The drawing under review shows one solid part. Ordinate dimensions are in mm from its lowest x, y, z. A direction names the side the tool comes from. Give positions to 0.01 mm unless a question says otherwise; leave off trailing zeros. Order: outer loops, then holes, each group sorted by start corner. A loop starts at its lowest first (then second) coordinate and runs counter-clockwise, first axis right, second up. Notation, with made-up numbers: (48.25, 39.25) - (62.25, 39.25) arc R22 cw to (62.25, 74.25) - close; hole circle Ø10 at (68.25, 12.25). An arc over 180 degrees is marked (long way). Answer as a JSON object with one key per item and string values. Group by question number.
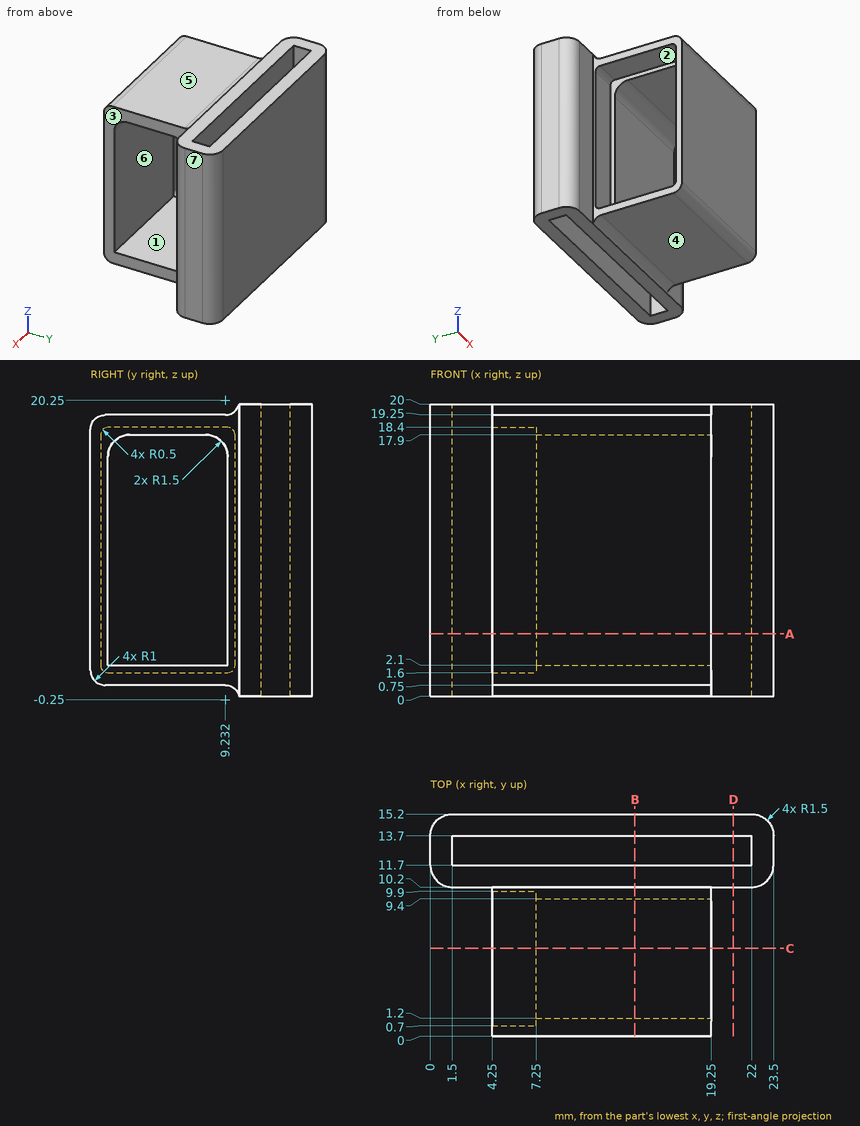
1) Consider section D-D (x = 20.75). Give the boundary of the cut face in (y, z), plus the area to 3 significant figures.
2) For line 1 (Y direction, x = 11, z = 5); line 2 (Z direction, x = 12.5, y = 3); line 3 (Y direction, x = 3, z = 16), list the stretches that pass through material, from the lowest coordinate up.
3) Consider section C-C (y = 6). Give the boundary of the cut face in (x, z), plus the area to 3 significant figures.
4) Consider section A-A (z = 4.25). Give the boundary of the cut face in (x, y), plus the area to 3 significant figures.
5) For pin 1 (8 mm diameter, centred on x = 4, y = 2, fed in from +Z); pin 2 (6 mm diameter, centred on y = 5, z = 17, fed in from -X); pin 3 (3 mm diameter, centred on x = 2.5, z = 14.5, fed in from -Y), all flat-tipped, find the tip position at first contact; note any pin that passes through.
6) Mouldability with a two-part tool opening along Z and no side actions: class the marked faces 4, 5, 6 and 7 as released by +Z, released by -Z, zero draft, split by the parting line, or undercut.
7) For the marked faces 1, 2 and 3, list the 3-axis set-ups (+Z, -Z, +X, -X, +Y, -Y) from which the entire face can be reached by the end or side of a thin tool; tool diameter is ignored.
8) Consider section B-B (x = 14). Give the boundary of the cut face in (y, z).
Result set:
{
 "1": {"outline": "(10.2, 0) - (11.7, 0) - (11.7, 20) - (10.2, 20) - close; (13.7, 0) - (15.2, 0) - (15.2, 20) - (13.7, 20) - close", "area": "60.0 mm2"},
 "2": {"line 1": "y = 0 to 1.2, 9.4 to 11.7, 13.7 to 15.2", "line 2": "z = 0.75 to 2.1, 17.9 to 19.25", "line 3": "y = 10.2 to 11.7, 13.7 to 15.2"},
 "3": {"outline": "(4.25, 0.75) - (19.25, 0.75) - (19.25, 2.1) - (7.25, 2.1) - (7.25, 1.6) - (4.25, 1.6) - close; (4.25, 18.4) - (7.25, 18.4) - (7.25, 17.9) - (19.25, 17.9) - (19.25, 19.25) - (4.25, 19.25) - close", "area": "37.5 mm2"},
 "4": {"outline": "(0, 11.7) arc R1.5 ccw to (1.5, 10.2) - (4.25, 10.2) - (4.25, 9.9) - (7.25, 9.9) - (7.25, 9.4) - (19.25, 9.4) - (19.25, 10.2) - (22, 10.2) arc R1.5 ccw to (23.5, 11.7) - (23.5, 13.7) arc R1.5 ccw to (22, 15.2) - (1.5, 15.2) arc R1.5 ccw to (0, 13.7) - close; (4.25, 0) - (19.25, 0) - (19.25, 1.2) - (7.25, 1.2) - (7.25, 0.7) - (4.25, 0.7) - close; hole (1.5, 11.7) - (22, 11.7) - (22, 13.7) - (1.5, 13.7) - close", "area": "102 mm2"},
 "5": {"pin 1": "stops at z = 19.25", "pin 2": "stops at x = 4.25", "pin 3": "stops at y = 10.2"},
 "6": {"face 4": "released by -Z", "face 5": "released by +Z", "face 6": "undercut", "face 7": "zero draft"},
 "7": {"face 1": "+X, -X", "face 2": "-X", "face 3": "+Z, -Z, +X, -Y"},
 "8": {"outline": "(0, 1.75) arc R1 ccw to (1, 0.75) - (9.23, 0.75) arc R1 cw to (10.2, 0) - (11.7, 0) - (11.7, 20) - (10.2, 20) arc R1 cw to (9.23, 19.25) - (1, 19.25) arc R1 ccw to (0, 18.25) - close; (13.7, 0) - (15.2, 0) - (15.2, 20) - (13.7, 20) - close; hole (1.2, 2.1) - (9.4, 2.1) - (9.4, 16.4) arc R1.5 ccw to (7.9, 17.9) - (2.7, 17.9) arc R1.5 ccw to (1.2, 16.4) - close"}
}
